Source: three-view drawing plus pictorial views. Frame: mm from the lowest corner of the part. Coordinates: 2 decimals unless noted, no trailing zeros. Order: outer loops, then holes, each group sorted by start corner. A loop starts at its lowest first (then second) coordinate and runs counter-clockwise, first axis right, second up. Notation, with made-up numbers: (34, 75.5) - (59, 75.5) arc R8 cw to (59, 79.5) - close; hole circle Ø3 at (-30, 70). An arc over 180 degrees is marked (long way). One line per question, with ' | ' between items.
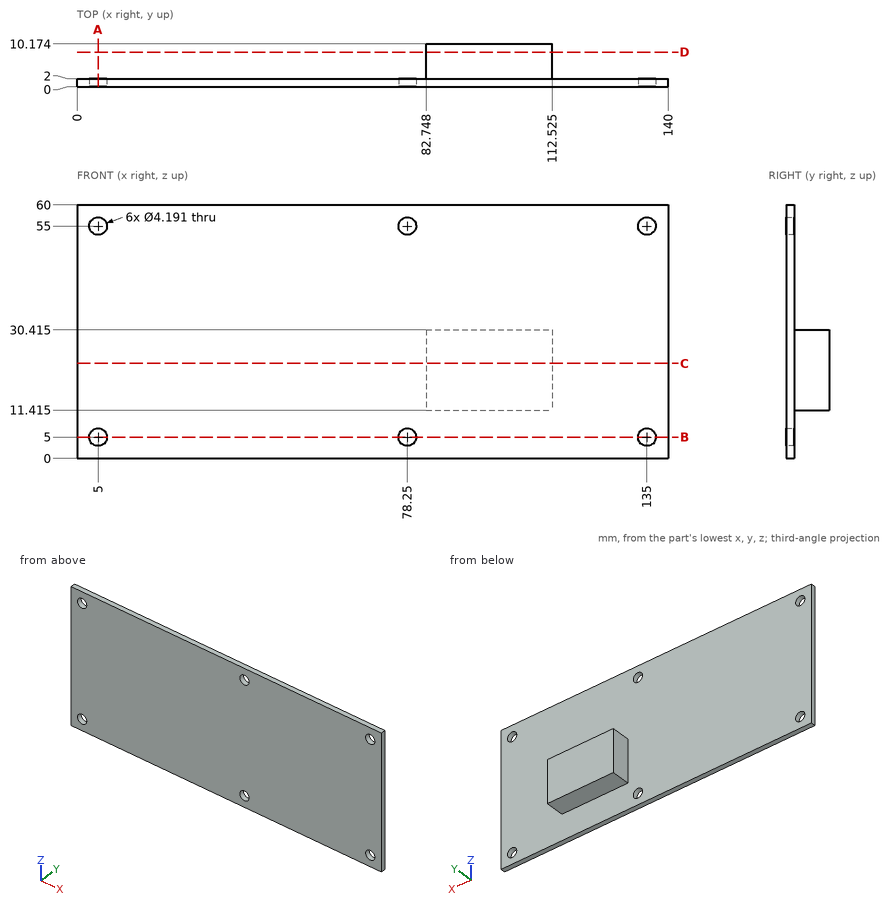
Item 1: Ray query, line 1 (X direction, y = 1.2, z = 55) (1 decimal); line 2 (Z direction, x = 135, y = 0.6) (1 decimal); line 3 (Y direction, x = 127, z = 23.5). Return the intervals inside material, ascending.
Data:
line 1: 0 to 2.9, 7.1 to 76.2, 80.3 to 132.9, 137.1 to 140 | line 2: 0 to 2.9, 7.1 to 52.9, 57.1 to 60 | line 3: 0 to 2
Item 2: Section C-C on z = 22.5. Return the cut outline in (x, y) (1 decimal).
Data:
outline: (0, 0) - (140, 0) - (140, 2) - (112.5, 2) - (112.5, 10.2) - (82.7, 10.2) - (82.7, 2) - (0, 2) - close
Item 3: Section B-B on z = 5. Return the cut outline in (x, y) (1 decimal).
Data:
outline: (0, 0) - (2.9, 0) - (2.9, 2) - (0, 2) - close; (7.1, 0) - (76.2, 0) - (76.2, 2) - (7.1, 2) - close; (80.3, 0) - (132.9, 0) - (132.9, 2) - (80.3, 2) - close; (137.1, 0) - (140, 0) - (140, 2) - (137.1, 2) - close
Item 4: Contact query for flat-ended pins moving along their axis: P1, Ø1, axis at y = 6.5, z = 25.5, coming from the -X side; P2, Ø5.5, axis at x = 78.25, z = 5, coming from the +Y side; P3, Ø4, axis at x = 96.5, y = 6, coming from the +Z side (1 decimal). Output: stop coordinate, or through.
Data:
P1: x = 82.75 | P2: y = 2 | P3: z = 30.4
Item 5: Section D-D on y = 8.25. Return the cut outline in (x, z) (1 decimal).
Data:
outline: (82.7, 11.4) - (112.5, 11.4) - (112.5, 30.4) - (82.7, 30.4) - close
Item 6: Section A-A on x = 5. Return the cut outline in (y, z) (1 decimal), and give its area (3 significant figures).
Data:
outline: (0, 0) - (2, 0) - (2, 2.9) - (0, 2.9) - close; (0, 7.1) - (2, 7.1) - (2, 52.9) - (0, 52.9) - close; (0, 57.1) - (2, 57.1) - (2, 60) - (0, 60) - close | area: 103 mm^2
